Verification items for the finished model (mm, model axes). Face numbers are marked on the shaded views. Coordinates: 2 decimals unless noted, no trailing zeros. Order: outer loops, then holes, each group sorted by start corner. A loop starts at its lowest first (then second) coordinate and runs counter-clockwise, first axis right, second up. Notation, with made-up numbers: M 8.25,36.5 L 41.25,36.5 A30 cw 41.25,60.5 Z; hole C 69.5,6.25 d5. An arc over 180 degrees is marked long. Return JSON: item names as keys, results as strings. Group by question number.
1. Section check A-A, the plane y = -6. Record the cut outline in (x, z), plus the area to 3 significant figures.
2. Gauge pin test, flat end, axial feed: pin 1 (2.5 mm diameter, centred on x = -8.5, z = 71, fed in from -Y). Record the tip position at first contact, or that the pin passes through.
3. Mould release check, pull along Y, two halves, no side actions. Record for the marked faces 1 and 2: +Y half, -Y half, draft (parallel to the pull), parting line (faces both ways), or undercut.
4. Material ranges on line 1 along Z through (x, y) = (-7, -8); line 2 along Z through (x, y) = (13, -2.75); line 3 along Z through (x, y) = (-4.5, -8.75), recorded low to high.
```python
from build123d import *

# Parameters (mm, degrees)
SKETCH1_W           = 50
SKETCH1_H           = 460
BOSS_EXTRUDE1_DEPTH = 10
CUT_EXTRUDE1_REACH  = 12
SKETCH2_R           = 2.75
SKETCH3_R           = 4.5
CUT_EXTRUDE2_DEPTH  = 5.5
CUT_EXTRUDE3_REACH  = 12
SKETCH4_R           = 2.75
SKETCH5_R           = 4.5
CUT_EXTRUDE4_DEPTH  = 5.5
FILLET2_R           = 4.5
CUT_EXTRUDE5_REACH  = 12
SKETCH6_R           = 3


with BuildPart() as part:
    # Sketch1 → Boss-Extrude1 (new body)
    with BuildSketch(Plane.XZ):
        with Locations((12.35332591, 254.692172039)):
            Rectangle(SKETCH1_W, SKETCH1_H)
    extrude(amount=BOSS_EXTRUDE1_DEPTH)

    # Sketch2 → Cut-Extrude1 (cut, up to next)
    with BuildSketch(Plane.XZ.offset(10), mode=Mode.PRIVATE) as cut_extrude1_sk1:
        with Locations((32.35332591, 69.692172039)):
            Circle(SKETCH2_R)
    cut_extrude1_tool1 = extrude(cut_extrude1_sk1.sketch, amount=-CUT_EXTRUDE1_REACH, mode=Mode.PRIVATE) & part.part
    add(cut_extrude1_tool1.solids().sort_by_distance((32.353326, -10, 69.692172))[0], mode=Mode.SUBTRACT)
    # Sketch2 → Cut-Extrude1 (cut, up to next)
    with BuildSketch(Plane.XZ.offset(10), mode=Mode.PRIVATE) as cut_extrude1_sk2:
        with Locations((-7.64667409, 69.692172039)):
            Circle(SKETCH2_R)
    cut_extrude1_tool2 = extrude(cut_extrude1_sk2.sketch, amount=-CUT_EXTRUDE1_REACH, mode=Mode.PRIVATE) & part.part
    add(cut_extrude1_tool2.solids().sort_by_distance((-7.646674, -10, 69.692172))[0], mode=Mode.SUBTRACT)
    # Sketch2 → Cut-Extrude1 (cut, up to next)
    with BuildSketch(Plane.XZ.offset(10), mode=Mode.PRIVATE) as cut_extrude1_sk3:
        with Locations((12.35332591, 49.692172039)):
            Circle(SKETCH2_R)
    cut_extrude1_tool3 = extrude(cut_extrude1_sk3.sketch, amount=-CUT_EXTRUDE1_REACH, mode=Mode.PRIVATE) & part.part
    add(cut_extrude1_tool3.solids().sort_by_distance((12.353326, -10, 49.692172))[0], mode=Mode.SUBTRACT)

    # Sketch3 → Cut-Extrude2 (cut)
    with BuildSketch(Plane.XZ.offset(10)):
        with Locations((-7.64667409, 69.692172039)):
            Circle(SKETCH3_R)
        with Locations((32.35332591, 69.692172039)):
            Circle(SKETCH3_R)
        with Locations((12.35332591, 49.692172039)):
            Circle(SKETCH3_R)
    extrude(amount=-CUT_EXTRUDE2_DEPTH, mode=Mode.SUBTRACT)

    # Sketch4 → Cut-Extrude3 (cut, up to next)
    with BuildSketch(Plane.XZ.offset(10), mode=Mode.PRIVATE) as cut_extrude3_sk1:
        with Locations((-7.64667409, 459.692172039)):
            Circle(SKETCH4_R)
    cut_extrude3_tool1 = extrude(cut_extrude3_sk1.sketch, amount=-CUT_EXTRUDE3_REACH, mode=Mode.PRIVATE) & part.part
    add(cut_extrude3_tool1.solids().sort_by_distance((-7.646674, -10, 459.692172))[0], mode=Mode.SUBTRACT)
    # Sketch4 → Cut-Extrude3 (cut, up to next)
    with BuildSketch(Plane.XZ.offset(10), mode=Mode.PRIVATE) as cut_extrude3_sk2:
        with Locations((32.35332591, 459.692172039)):
            Circle(SKETCH4_R)
    cut_extrude3_tool2 = extrude(cut_extrude3_sk2.sketch, amount=-CUT_EXTRUDE3_REACH, mode=Mode.PRIVATE) & part.part
    add(cut_extrude3_tool2.solids().sort_by_distance((32.353326, -10, 459.692172))[0], mode=Mode.SUBTRACT)

    # Sketch5 → Cut-Extrude4 (cut)
    with BuildSketch(Plane.XZ.offset(10)):
        with Locations((-7.64667409, 459.692172039)):
            Circle(SKETCH5_R)
        with Locations((32.35332591, 459.692172039)):
            Circle(SKETCH5_R)
    extrude(amount=-CUT_EXTRUDE4_DEPTH, mode=Mode.SUBTRACT)

    # Fillet2
    fillet2_edges = [part.edges().sort_by_distance(p)[0] for p in [
        (37.35332591, -5, 24.692172039),
        (-12.64667409, -5, 24.692172039),
        (-12.64667409, -5, 484.692172039),
        (37.35332591, -5, 484.692172039),
    ]]
    fillet(fillet2_edges, radius=FILLET2_R)

    # Sketch6 → Cut-Extrude5 (cut, up to next)
    with BuildSketch(Plane(origin=(0, 0, 0), x_dir=(-1, 0, 0), z_dir=(0, 1, 0)), mode=Mode.PRIVATE) as cut_extrude5_sk1:
        with Locations((-12.35332591, 474.692172039)):
            Circle(SKETCH6_R)
    cut_extrude5_tool1 = extrude(cut_extrude5_sk1.sketch, amount=-CUT_EXTRUDE5_REACH, mode=Mode.PRIVATE) & part.part
    add(cut_extrude5_tool1.solids().sort_by_distance((12.353326, 0, 474.692172))[0], mode=Mode.SUBTRACT)
    # Sketch6 → Cut-Extrude5 (cut, up to next)
    with BuildSketch(Plane(origin=(0, 0, 0), x_dir=(-1, 0, 0), z_dir=(0, 1, 0)), mode=Mode.PRIVATE) as cut_extrude5_sk2:
        with Locations((-12.35332591, 34.692172039)):
            Circle(SKETCH6_R)
    cut_extrude5_tool2 = extrude(cut_extrude5_sk2.sketch, amount=-CUT_EXTRUDE5_REACH, mode=Mode.PRIVATE) & part.part
    add(cut_extrude5_tool2.solids().sort_by_distance((12.353326, 0, 34.692172))[0], mode=Mode.SUBTRACT)


solid = part.part
```
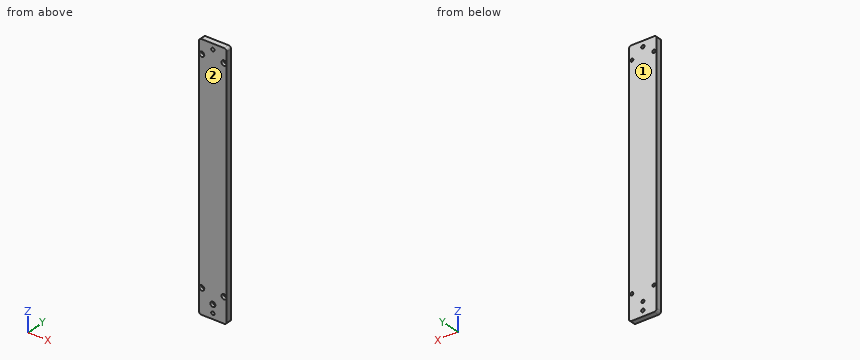
Answers follow:
{
 "1": {"outline": "M -12.65,29.19 A4.5 ccw -8.15,24.69 L 32.85,24.69 A4.5 ccw 37.35,29.19 L 37.35,480.19 A4.5 ccw 32.85,484.69 L -8.15,484.69 A4.5 ccw -12.65,480.19 Z; hole C -7.65,69.69 d9; hole C -7.65,459.69 d9; hole C 12.35,49.69 d9; hole C 12.35,34.69 d6; hole C 12.35,474.69 d6; hole C 32.35,69.69 d9; hole C 32.35,459.69 d9", "area": "22,600 mm^2"},
 "2": {"pin 1": "y = -4.5"},
 "3": {"face 1": "+Y half", "face 2": "-Y half"},
 "4": {"line 1": "24.69 to 65.24, 74.15 to 455.24, 464.15 to 484.69", "line 2": "24.69 to 31.76, 37.62 to 47.02, 52.37 to 471.76, 477.62 to 484.69", "line 3": "24.69 to 66.48, 72.91 to 456.48, 462.91 to 484.69"}
}
